Geometry: see drawing. Coordinates: mm, zero at the bounding-box minimum. A direction names the side the tool comes from. Give positions to 0.01 mm unless a question says otherwise; leave off trailing zeros. Loops run counter-clockwise (first coordinate to the right, second up) from the corner with the lowest first, then second, coordinate; pieces in that order, holes last. Notation, with made-up numbers: M 85,-21.5 L 114,-21.5 A34 cw 114,9.5 Z; hole C 12,41.25 d2. An arc over 180 degrees is marked long. Answer in a Markdown table with one row per item.
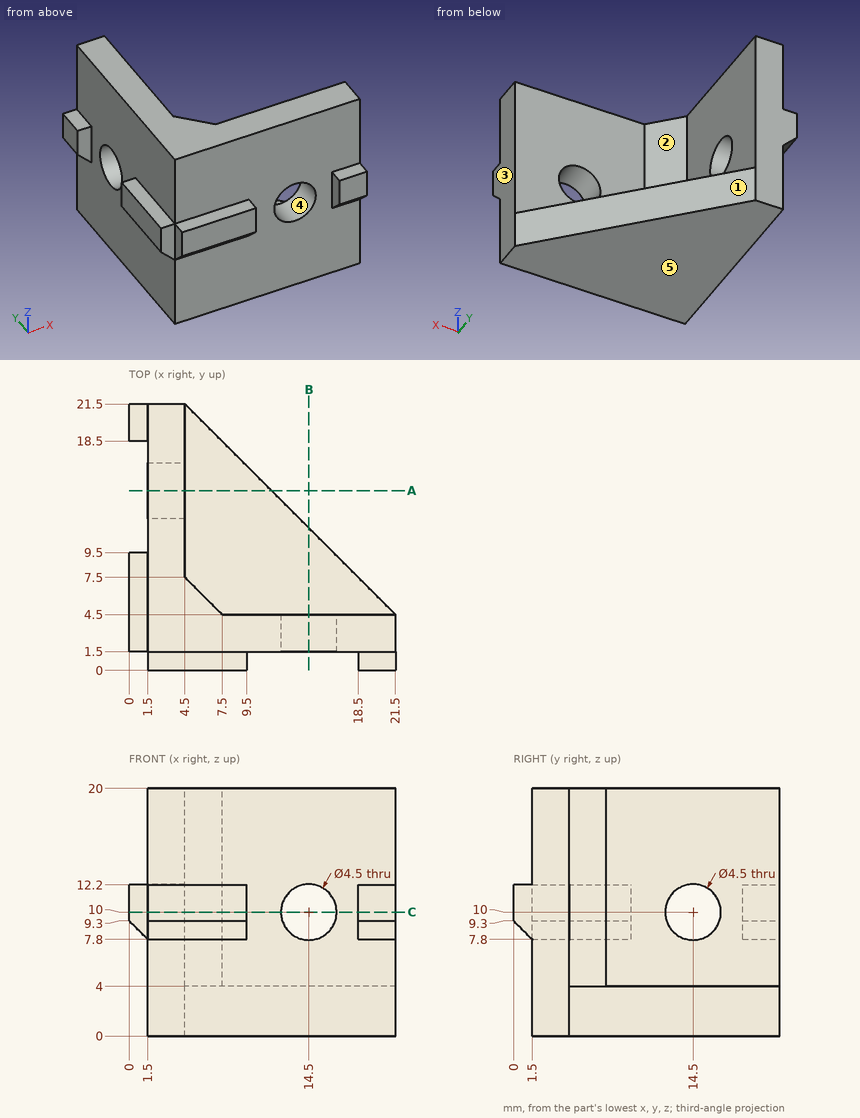
1) Set-up query: the marked faces 1 and 2. Return all of +Z, -Z, +X, -X, +Y, -Y with unobstructed straight access to the full face (end or side cutting, diameter ignored); none if empty.
Reply:
| item | result |
|---|---|
| face 1 | +Z, -Z, +X, +Y |
| face 2 | +Z, +X, +Y |
2) Section C-C, the plane z = 10. Return loops of the section in (x, y).
Reply:
| item | result |
|---|---|
| outline | M 0,1.5 L 1.5,1.5 L 1.5,0 L 9.5,0 L 9.5,1.5 L 12.25,1.5 L 12.25,4.5 L 7.5,4.5 L 4.5,7.5 L 4.5,12.25 L 1.5,12.25 L 1.5,9.5 L 0,9.5 Z; M 0,18.5 L 1.5,18.5 L 1.5,16.75 L 4.5,16.75 L 4.5,21.5 L 0,21.5 Z; M 16.75,1.5 L 18.5,1.5 L 18.5,0 L 21.5,0 L 21.5,4.5 L 16.75,4.5 Z |
3) Material intervals for L1, parallel to Z at x = 2.95, y = 14.5; L2, parallel to X at y = 11.75, z = 10.5, sorted ascending.
Reply:
| item | result |
|---|---|
| L1 | z = 0 to 7.75, 12.25 to 20 |
| L2 | x = 1.5 to 4.5 |
4) Section A-A, the plane y = 14.5. Return loops of the section in (x, z).
Reply:
| item | result |
|---|---|
| outline | M 1.5,0 L 11.5,0 L 11.5,4 L 4.5,4 L 4.5,7.75 L 1.5,7.75 Z; M 1.5,12.25 L 4.5,12.25 L 4.5,20 L 1.5,20 Z |
5) Pull-direction query (X, two-part tool) for the marked faces 3, 4 and 5; classes: released by +X, released by -X, zero draft, split by the parting line, or undercut.
Reply:
| item | result |
|---|---|
| face 3 | released by +X |
| face 4 | undercut |
| face 5 | zero draft |
6) Pin query (flat end, axial travel): pin 1 Ø1.2 at (y, z) = (1, 9.5) entering from -X; pin 2 Ø1.6 at (x, y) = (19.5, 0.5) entering from +Z; pin 3 Ø1.5 at (x, z) = (5.5, 7) entering from -Y; pin 4 Ø1 at (y, z) = (18.5, 3) entering from +X. Return the tip coordinate at first contact, or that it passes through.
Reply:
| item | result |
|---|---|
| pin 1 | stops at x = 0 |
| pin 2 | stops at z = 12.2 |
| pin 3 | stops at y = 1.5 |
| pin 4 | stops at x = 8 |
